Geometry: see drawing. Coordinates: mm, zero at the bounding-box minimum. A direction names the side the tool comes from. Give positions to 0.01 mm unless a question says otherwise; leave off trailing zeros. Order: outer loops, then holes, each group sorted by start corner. A loop starts at its lowest first (then second) coordinate and runs counter-clockwise, first axis right, second up. Notation, with made-up numbers: (-13.5, -18) - (36.5, -18) arc R16 ccw to (36.5, 2) - close; hole circle Ø9 at (-4, 26.25). An arc over 180 degrees is marked (long way). Put each result on its own line as item: value. Start each with the question number.
1. Ray query, line 1 along Z through (x, y) = (3, 14.25) (1 decimal); line 2 along X through (y, z) = (15.25, 3.75) (1 decimal); line 3 along X through (y, z) = (11, 5.25) (1 decimal). Return the intervals inside material, ascending. Write a range as from..to.
2. Mould query, pull axis Y, two halves, no side actions, for the marked faces 1, 2 and 3. Classes: pulls with the +Y half, pulls with the -Y half, needs draft (parallel to the pull), parting line crosses it, or undercut.
3. First-contact query: P1, Ø0.5, axis at y = 0, z = 5.5, coming from the +X side; P2, Ø0.6, axis at x = 21, z = 6.5, coming from the -Y side (1 decimal); P3, Ø0.7, axis at y = 0, z = 3, coming from the -X side (1 decimal). Flat tips, straight axial feed; report the tip coordinate or a pass-through.
4. Section A-A on z = 5.5. Return the cut outline in (x, y) (1 decimal), plus the area to 3 significant figures.
5. Set-up query: the marked faces 4, 5 and 6. Return all of +Z, -Z, +X, -X, +Y, -Y with unobstructed straight access to the full face (end or side cutting, diameter ignored); none if empty.
6. Section D-D on z = 1. Return the cut outline in (x, y) (1 decimal).
7. Section C-C on y = 10.25. Return the cut outline in (x, z) (1 decimal).
8. Section B-B on x = 3.5. Return the cut outline in (y, z) (1 decimal), plus the area to 3 significant figures.
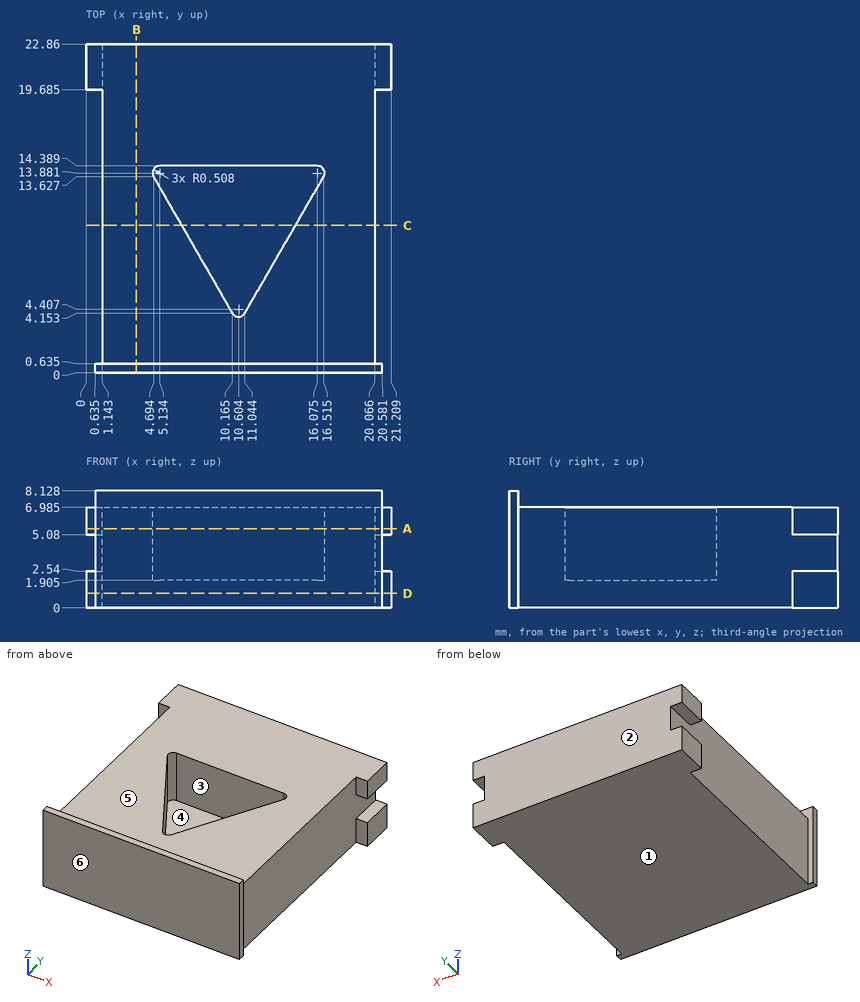
Resolved:
1. line 1: 0..7
1. line 2: 1.1..20.1
1. line 3: 1.1..6.2, 15..20.1
2. face 1: needs draft
2. face 2: pulls with the +Y half
2. face 3: undercut
3. P1: x = 20.58
3. P2: y = 19.7
3. P3: x = 0.6
4. outline: (0, 19.7) - (1.1, 19.7) - (1.1, 0.6) - (0.6, 0.6) - (0.6, 0) - (20.6, 0) - (20.6, 0.6) - (20.1, 0.6) - (20.1, 19.7) - (21.2, 19.7) - (21.2, 22.9) - (0, 22.9) - close; hole (4.7, 13.6) - (10.2, 4.2) arc R0.5 ccw to (11, 4.2) - (16.5, 13.6) arc R0.5 ccw to (16.1, 14.4) - (5.1, 14.4) arc R0.5 ccw to start
4. area: 371 mm^2
5. face 4: +Z
5. face 5: +Z, +X, -X, +Y
5. face 6: +Z, -Z, +X, -X, -Y
6. outline: (0, 19.7) - (1.1, 19.7) - (1.1, 0.6) - (0.6, 0.6) - (0.6, 0) - (20.6, 0) - (20.6, 0.6) - (20.1, 0.6) - (20.1, 19.7) - (21.2, 19.7) - (21.2, 22.9) - (0, 22.9) - close
7. outline: (1.1, 0) - (20.1, 0) - (20.1, 7) - (14.6, 7) - (14.6, 1.9) - (6.6, 1.9) - (6.6, 7) - (1.1, 7) - close
8. outline: (0, 0) - (22.9, 0) - (22.9, 7) - (0.6, 7) - (0.6, 8.1) - (0, 8.1) - close
8. area: 160 mm^2
